The figure shows three views and two pictorial views of one solid part (mm, origin at its lowest corner). Answer the questions. A direction names the side the tool comes from. Coordinates: 2 decimals unless noted, no trailing zeros. Loops run counter-clockwise (first coordinate to the right, second up) from the corner with the lowest first, then second, coordinate; pieces in that order, holes last. Notation, with made-up numbers: M 51.5,-13.5 L 68.5,-13.5 A24 cw 68.5,2.5 Z; hole C -10.5,20 d1. An arc over 180 degrees is marked long. One line per item, written item: value. Start each with the question number.
1. For the marked faces 1 and 2, determine the directions among +Z, -Z, +X, -X, +Y, -Y from which every point of the face is accessible in a straight line to the end or side of a thin tool.
2. The part is cut by section C-C (y = 11.5). Write down the section's boundary in (x, z) (3 decimals), then the cut area to 3 significant figures.
3. The part is cut by section B-B (z = 6). Write down the section's boundary in (x, y) (3 decimals), then the cut area to 3 significant figures.
4. Flat-ended cylindrical pins translate along their axes: pin 1 (5 mm diameter, centred on x = 32, y = 7.5, fed in from -Z) (3 decimals); pin 2 (3 mm diameter, centred on y = 6, z = 3.5, fed in from -X); pin 3 (2 mm diameter, centred on x = 10, z = 1.5, fed in from +Y) (3 decimals). Find the tip coordinate at first contact, or state that the pin passes through.
5. The part is cut by section A-A (x = 45). Write down the section's boundary in (y, z) (3 decimals), then the cut area to 3 significant figures.
6. Consider probe 1 along Z at (x, y) = (36, 5.5) (3 decimals); probe 2 along Y at (x, z) = (54.5, 9) (3 decimals). Determine where each line is inside the solid, lowest interval first.
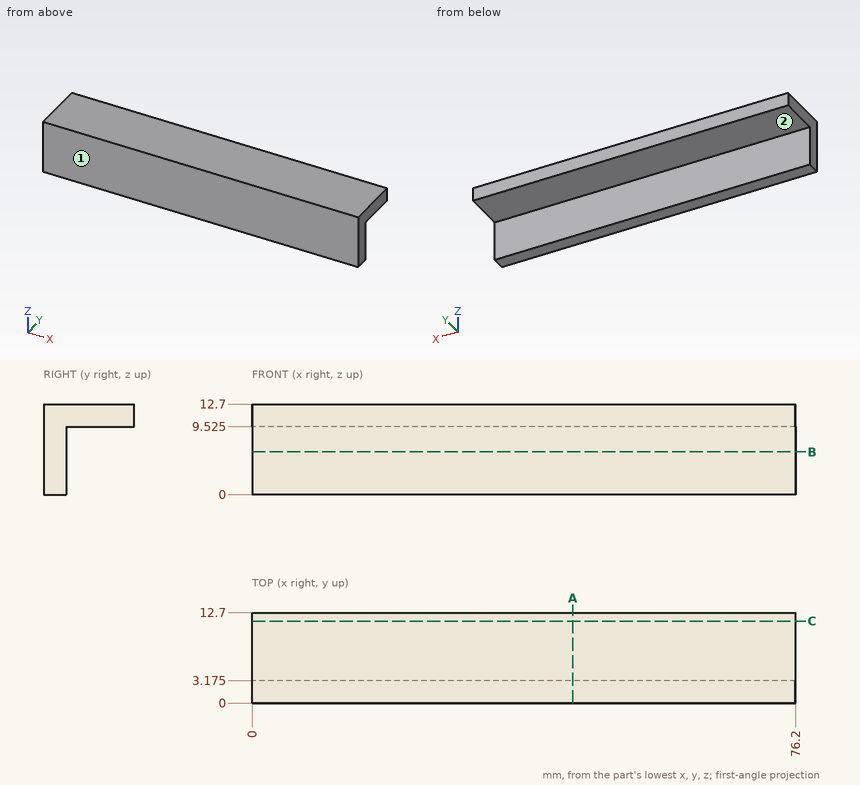
Answer block:
1. face 1: +Z, -Z, +X, -X, -Y
1. face 2: -Z, +X, -X, +Y
2. outline: M 0,9.525 L 76.2,9.525 L 76.2,12.7 L 0,12.7 Z
2. area: 242 mm2
3. outline: M 0,0 L 76.2,0 L 76.2,3.175 L 0,3.175 Z
3. area: 242 mm2
4. pin 1: stops at z = 9.525
4. pin 2: passes through
4. pin 3: stops at y = 3.175
5. outline: M 0,0 L 3.175,0 L 3.175,9.525 L 12.7,9.525 L 12.7,12.7 L 0,12.7 Z
5. area: 70.6 mm2
6. probe 1: z = 9.525 to 12.7
6. probe 2: y = 0 to 3.175
